Autodesk Inventor part; units mm, degrees
sketch "Skizze1" plane through (0, 0, 0) normal (0, 1, 0) x (-1, 0, 0)
  circle A0 centre (0, 0) radius 20
  circle A1 centre (0, 0) radius 26
  dimension "d0" = 40
  dimension "d1" = 52
extrude "Extrusion1" add sketch "Skizze1" along normal blind 9
chamfer "Fase1" distance 3 angle 45 1 edges at (26, 9, 0)
sketch "Skizze2" plane through (0, 9, 0) normal (0, 1, 0) x (1, 0, 0)
  line L0 (-28.5, -3) -> (-23.5, -3)
  line L1 (-23.5, -3) -> (-23.5, 3)
  line L2 (-23.5, 3) -> (-28.5, 3)
  line L3 (-28.5, 3) -> (-28.5, -3)
  circle A0 centre (0, 0) radius 26
  line L4 (-28.5, -3) -> (-23.5, 3) construction
  line L5 (-23.5, -3) -> (-28.5, 3) construction
  line L6 (3, 23.5) -> (-3, 23.5)
  line L7 (-3, 23.5) -> (-3, 28.5)
  line L8 (-3, 28.5) -> (3, 28.5)
  line L9 (3, 28.5) -> (3, 23.5)
  line L10 (3, 23.5) -> (-3, 28.5) construction
  line L11 (-3, 23.5) -> (3, 28.5) construction
  line L12 (3, -23.5) -> (-3, -23.5)
  line L13 (-3, -23.5) -> (-3, -28.5)
  line L14 (-3, -28.5) -> (3, -28.5)
  line L15 (3, -28.5) -> (3, -23.5)
  line L16 (3, -23.5) -> (-3, -28.5) construction
  line L17 (-3, -23.5) -> (3, -28.5) construction
  line L18 (23.5, -3) -> (28.5, -3)
  line L19 (28.5, -3) -> (28.5, 3)
  line L20 (28.5, 3) -> (23.5, 3)
  line L21 (23.5, 3) -> (23.5, -3)
  line L22 (23.5, -3) -> (28.5, 3) construction
  line L23 (28.5, -3) -> (23.5, 3) construction
  line L24 (-39.9, 0) -> (39.9, 0)
  point P0 (-26, 0)
  point P1 (0, 26)
  point P2 (0, -26)
  point P3 (26, 0)
  dimension "d7" = 5
  dimension "d8" = 6
  dimension "d9" = 5
  dimension "d10" = 26
  dimension "d11" = 6
  dimension "d12" = 0
  dimension "d13" = 6
  dimension "d14" = 5
  dimension "d15" = 5
  dimension "d16" = 0
extrude "Extrusion2" cut sketch "Skizze2" against normal blind 9 contours L3 L24 A0 L0 | A0 L24 L1 L0 | L3 L2 A0 L24 | A0 L2 L1 L24 | L13 L12 L15 A0 | A0 L15 L14 L13 | L24 A0 L18 L21 | L21 L20 A0 L24 | L7 L8 L9 A0 | A0 L9 L6 L7 | A0 L24 L19 L18 | A0 L20 L19 L24
thread "Gewinde1"
properties part number "Sicherheitsmutter_m40"
Input: part model. Units: mm. Frame: model coordinates. A direction names the side the tool comes from. Give positions to 0.01 mm unless a question says otherwise; leave off trailing zeros. Order: outer loops, then holes, each group sorted by start corner. A loop starts at its lowest first (then second) coordinate and runs counter-clockwise, first axis right, second up. Notation, with made-up numbers: M 78,37.5 L 86,37.5 A19 cw 86,47.5 Z; hole C -14.5,36.25 d3. An arc over 180 degrees is marked long. One line per question, with ' | ' between items. Start each with the question number.
1. Section query B-B (z = 0). Return the cut outline in (x, y), and give its area (4 significant figures).
2. Access query for faces 1 (the face through (-23.5, 4, 0)), 2 (the face through (-18.56, 2.96, -18.21)), 3 (the face through (-3, 3, -25)), 4 (the face through (25, 3, -3)). Directions: +Z, -Z, +X, -X, +Y, -Y. A direction counts if a zero-diameter tool reaches every point of the face in a straight line with its end or side. Return the directions, or none.
3. First-contact query: pin 1 Ø3 at (x, y) = (-17.5, 3) entering from +Z; pin 2 Ø2.5 at (y, z) = (2.5, -25) entering from +X; pin 3 Ø1 at (y, z) = (2, 7) entering from +X. Flat tips, straight axial feed; report the tip coordinate or a pass-through.
4. Section query C-C (y = 4). Return the cut outline in (x, z), and give its area (3 significant figures).
5. Section query A-A (x = 0). Return the cut outline in (y, z), and give its area (4 significant figures).
6. Pull-direction query (Z, two-part tool) for faces 5 (the face through (0, 4, -23.5)), 6 (the face through (3, 3, 25)), 7 (the face through (23.5, 4, 0)), 8 (the face through (0, 4, 23.5)); classes: released by +Z, released by -Z, zero draft, split by the parting line, or undercut.
7. Material intervals for probe 1 along Z at (x, y) = (0, 6.5); probe 2 along X at (y, z) = (3.5, -7) (3 decimals); probe 3 along Z at (x, y) = (10.5, 5.75), sorted ascending. Write a range as [from, to].
8. Section query D-D (y = 7.25). Return the cut outline in (x, z), and give its area (3 significant figures).
Here are the results:
1) outline: M -23.5,0 L -20,0 L -20,9 L -23,9 L -23.5,8.5 Z; M 20,0 L 23.5,0 L 23.5,8.5 L 23,9 L 20,9 Z | area: 62.75 mm²
2) face 1: -X, +Y, -Y | face 2: -Z, -X, +Y, -Y | face 3: -Z, +Y, -Y | face 4: +X, +Y, -Y
3) pin 1: z = 20.49 | pin 2: x = 10.58 | pin 3: x = 25.17
4) outline: M -25.83,-3 A26 ccw -3,-25.83 L -3,-23.5 L 3,-23.5 L 3,-25.83 A26 ccw 25.83,-3 L 23.5,-3 L 23.5,3 L 25.83,3 A26 ccw 3,25.83 L 3,23.5 L -3,23.5 L -3,25.83 A26 ccw -25.83,3 L -23.5,3 L -23.5,-3 Z; hole C 0,0 d40 | area: 808 mm²
5) outline: M 0,-23.5 L 8.5,-23.5 L 9,-23 L 9,-20 L 0,-20 Z; M 0,20 L 9,20 L 9,23 L 8.5,23.5 L 0,23.5 Z | area: 62.75 mm²
6) face 5: released by -Z | face 6: zero draft | face 7: undercut | face 8: released by +Z
7) probe 1: [-23.5, -20], [20, 23.5] | probe 2: [-25.04, -18.735], [18.735, 25.04] | probe 3: [-23.79, -17.02], [17.02, 23.79]
8) outline: M -24.57,-3 A24.75 ccw -3,-24.57 L -3,-23.5 L 3,-23.5 L 3,-24.57 A24.75 ccw 24.57,-3 L 23.5,-3 L 23.5,3 L 24.57,3 A24.75 ccw 3,24.57 L 3,23.5 L -3,23.5 L -3,24.57 A24.75 ccw -24.57,3 L -23.5,3 L -23.5,-3 Z; hole C 0,0 d40 | area: 639 mm²
